Part model, mm, in its own coordinate system. Face numbers are marked on the shaded views. A direction names the side the tool comes from. Give positions to 0.01 mm unless a question says otherwise; leave off trailing zeros. Write each loop counter-clockwise with the first axis right and the second up, starting at its lowest first coordinate (ties: lowest second). Pieces come first, ordered by that corner, then holes.
Autodesk Inventor part; units mm, degrees
ref_plane "Work Plane1" through (0, 0, 0) normal (0, 0, 1) x (1, 0, 0)
ref_plane "Work Plane2" through (0, -215, -35.5) normal (0, 0, -1) x (-1, 0, 0)
ref_plane "YZ Plane" through (0, 0, 0) normal (1, 0, 0) x (0, 1, 0)
ref_plane "Work Plane1" through (0, 0, 0) normal (0, 0, 1) x (1, 0, 0)
sketch "Sketch1" plane through (0, 0, 0) normal (0, 0, 1) x (1, 0, 0)
  line L0 (0, 0) -> (77.47, 0)
  line L1 (77.47, 0) -> (77.47, -114.3)
  line L2 (77.47, -114.3) -> (0, -114.3)
  line L3 (0, -114.3) -> (0, 0)
  circle A0 centre (56.1975, -55.5625) radius 4.8895
  circle A1 centre (4.4958, -6.5024) radius 1.7
  circle A2 centre (4.4958, -35.9918) radius 1.7
  circle A3 centre (4.4958, -83.9978) radius 1.7
  dimension "d0" = 77.47
  dimension "d1" = 114.3
  dimension "d2" = 9.779
  dimension "d42" = 3.4
  dimension "d43" = 6.5024
  dimension "d44" = 4.4958
  dimension "d53" = 3.4
  dimension "d54" = 35.9918
  dimension "d55" = 4.4958
  dimension "d56" = 3.4
  dimension "d57" = 83.9978
  dimension "d58" = 4.4958
  dimension "d64" = 56.1975
extrude "Servo Mount Side" add sketch "Sketch1" along normal blind 2.54
ref_plane "Work Plane2" through (0, -215, -35.5) normal (0, 0, -1) x (-1, 0, 0)
sketch "Sketch3" plane through (0, -215, -35.5) normal (0, 0, -1) x (-1, 0, 0)
  line L0 (-77.47, 215) -> (0, 215)
  line L1 (0, 215) -> (-77.47, 215)
  line L2 (-77.47, 215) -> (-77.47, 100.7)
  line L3 (-77.47, 100.7) -> (0, 100.7)
  line L4 (0, 100.7) -> (0, 215)
  circle A0 centre (-56.1975, 159.4375) radius 4.8895
  circle A1 centre (-4.4958, 204.6622) radius 1.7
  circle A2 centre (-4.4958, 179.0082) radius 1.7
  circle A3 centre (-4.4958, 131.0022) radius 1.7
  circle A4 centre (-20, 202) radius 1.7
  circle A5 centre (-4.4958, 167.9084) radius 1.7
  dimension "d13" = 114.3
  dimension "d14" = 77.47
  dimension "d48" = 3.4
  dimension "d49" = 10.3378
  dimension "d50" = 4.4958
  dimension "d51" = 3.4
  dimension "d52" = 3.4
  dimension "d59" = 35.9918
  dimension "d60" = 83.9978
  dimension "d61" = 4.4958
  dimension "d62" = 4.4958
  dimension "d65" = 3.4
  dimension "d66" = 20
  dimension "d67" = 13
  dimension "d68" = 3.4
  dimension "d69" = 11.0998
  dimension "d70" = 4.4958
extrude "Encoder Mount Side" add sketch "Sketch3" along normal blind 2.54
sketch "Sketch4" plane through (0, -215, -35.5) normal (0, 0, 1) x (1, 0, 0)
  line L0 (77.47, 100.7) -> (0, 100.7)
  line L1 (10.033, 100.7) -> (29.083, 100.7)
  line L2 (29.083, 100.7) -> (29.083, 110.225)
  line L3 (29.083, 110.225) -> (10.033, 110.225)
  line L4 (10.033, 110.225) -> (10.033, 100.7)
  line L5 (77.47, 100.7) -> (58.42, 100.7)
  line L6 (58.42, 100.7) -> (58.42, 110.225)
  line L7 (58.42, 110.225) -> (77.47, 110.225)
  line L8 (77.47, 110.225) -> (77.47, 100.7)
  line L9 (0, 100.7) -> (0, 215)
  dimension "d20" = 19.05
  dimension "d21" = 9.525
  dimension "d22" = 19.05
  dimension "d23" = 9.525
  dimension "d63" = 10.033
extrude "Extrusion3" add sketch "Sketch4" along normal up to surface (35.5 mm away)
sketch "Sketch5" plane through (0, -215, -38.04) normal (0, 0, -1) x (-1, 0, 0)
  circle A0 centre (-65.7225, 159.4375) radius 1.397
  circle A1 centre (-56.1975, 159.4375) radius 4.8895
  circle A2 centre (-62.9327, 152.7023) radius 1.397
  circle A3 centre (-56.1975, 149.9125) radius 1.397
  circle A4 centre (-49.4623, 152.7023) radius 1.397
  circle A5 centre (-46.6725, 159.4375) radius 1.397
  circle A6 centre (-49.4623, 166.1727) radius 1.397
  circle A7 centre (-56.1975, 168.9625) radius 1.397
  circle A8 centre (-62.9327, 166.1727) radius 1.397
  point P0 (0, 215)
  dimension "d26" = 2.794
  dimension "d27" = 9.525
  dimension "d30" = 360
extrude "Extrusion4" cut sketch "Sketch5" against normal blind 2.54
sketch "Sketch7" plane through (0, 0, 0) normal (0, 0, -1) x (-1, 0, 0)
  circle A0 centre (-49.4623, -62.2977) radius 1.397
  circle A1 centre (-49.4623, -48.8273) radius 1.397
  circle A2 centre (-65.7225, -55.5625) radius 1.397
  circle A3 centre (-46.6725, -55.5625) radius 1.397
  circle A4 centre (-62.9327, -48.8273) radius 1.397
  circle A5 centre (-62.9327, -62.2977) radius 1.397
  circle A6 centre (-56.1975, -65.0875) radius 1.397
  circle A7 centre (-56.1975, -46.0375) radius 1.397
  line L0 (0, -114.3) -> (0, 0)
  line L1 (0, 0) -> (-77.47, 0)
  line L2 (-77.47, 0) -> (-77.47, -114.3)
  line L3 (-77.47, -114.3) -> (0, -114.3)
  circle A8 centre (-56.1975, -55.5625) radius 4.8895
  circle A9 centre (-69.3421, -42.0921) radius 1.3525 construction
  circle A10 centre (-23.3529, -42.0921) radius 1.3525 construction
  circle A11 centre (-23.3529, -69.0329) radius 1.3525 construction
  circle A12 centre (-69.3421, -69.0329) radius 1.3525 construction
  circle A13 centre (-69.3421, -69.0329) radius 1.9304
  circle A14 centre (-69.3421, -42.0921) radius 1.9304
  circle A15 centre (-23.3529, -42.0921) radius 1.9304
  circle A16 centre (-23.3529, -69.0329) radius 1.9304
  dimension "d34" = 3.8608
  dimension "d35" = 3.8608
  dimension "d36" = 3.8608
  dimension "d37" = 3.8608
extrude "Extrusion5" cut sketch "Sketch7" against normal through all contours A13 | A14 | A15 | A16
sketch "Sketch8" plane through (0, 0, 2.54) normal (0, 0, 1) x (1, 0, 0)
  circle A0 centre (56.1975, -55.5625) radius 4.8895
  circle A1 centre (56.1975, -55.5625) radius 44.45
  point P0 (0, 0)
  dimension "d40" = 88.9
fillet "Fillet1" radius 50.8 2 edges at (77.47, 0, -36.77) (77.47, 0, 1.27)
equation "\"d55\" = d44"
equation "\"d58\" = d44"
equation "\"d13\" = d1"
equation "\"d14\" = d0"
equation "\"d50\" = d44"
equation "\"d61\" = d44"
equation "\"d62\" = d44"
equation "\"d70\" = d50"
properties part number "whole servo mount"
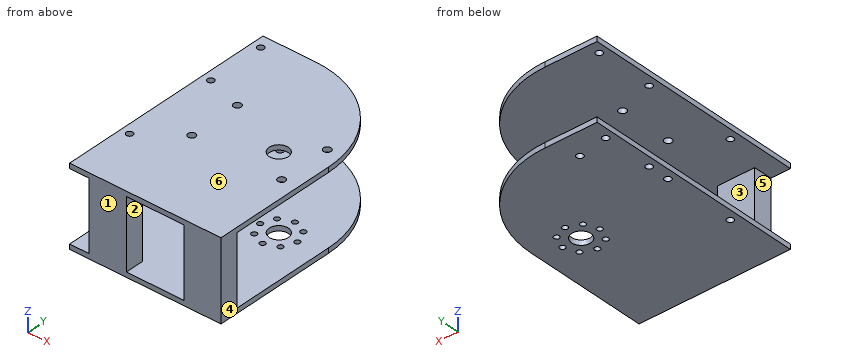
1) Two-plate mould, pull along Z, no slides. Class the marked faces 4, 5 and 6: +Z half, -Z half, draft (parallel to the pull), parting line (faces both ways), or undercut.
Answers follow:
face 4: draft
face 5: undercut
face 6: +Z half
2) Saw through at A-A, the plane y = -76.5. Write the cut outline in (x, z), then the cut area to 3 significant figures.
Answers follow:
outline: (0, -38.04) - (77.47, -38.04) - (77.47, -35.5) - (0, -35.5) - close; (0, 0) - (77.47, 0) - (77.47, 2.54) - (0, 2.54) - close
area: 394 mm2
3) Pin check, flat tips, straight feed: pin 1 Ø6 at (y, z) = (-101, -27.5) entering from -X; pin 2 Ø5 at (y, z) = (-108.5, -11) entering from -X; pin 3 Ø10 at (x, z) = (58.5, -13) entering from +Y (3 decimals); pin 4 Ø1.7 at (x, y) = (56.2, -65.09) entering from -Z. Stop position of each tip, or through.
Answers follow:
pin 1: passes through
pin 2: stops at x = 10.03
pin 3: stops at y = -104.775
pin 4: stops at z = 0
4) Saw through at C-C, the plane z = -17. Write the cut outline in (x, y) (3 decimals).
Answers follow:
outline: (10.033, -114.3) - (29.083, -114.3) - (29.083, -104.775) - (10.033, -104.775) - close; (58.42, -114.3) - (77.47, -114.3) - (77.47, -104.775) - (58.42, -104.775) - close
5) 3-axis set-ups, long thin cutter, end or side, ignore diameter. For the marked faces 1, 2 and 3: which of +Z, -Z, +X, -X, +Y, -Y reach the whole face in a straight line?
Answers follow:
face 1: +Z, -Z, +X, -X, -Y
face 2: +Y, -Y
face 3: +X, -X, +Y
6) Saw through at B-B, the plane x = 20. Write the cut outline in (y, z) (3 decimals).
Answers follow:
outline: (-114.3, -38.04) - (-14.7, -38.04) - (-14.7, -35.5) - (-104.775, -35.5) - (-104.775, 0) - (0, 0) - (0, 2.54) - (-114.3, 2.54) - close; (-11.3, -38.04) - (0, -38.04) - (0, -35.5) - (-11.3, -35.5) - close
7) Wall check: L1, parallel to Z at x = 22, y = -82; L2, parallel to Y at x = 20, z = -36; L3, parallel to Y at x = 59.5, z = -1.5 (3 decimals). Give the ranges that are in metal, low to high.
Answers follow:
L1: z = -38.04 to -35.5, 0 to 2.54
L2: y = -114.3 to -14.7, -11.3 to 0
L3: y = -114.3 to -104.775
